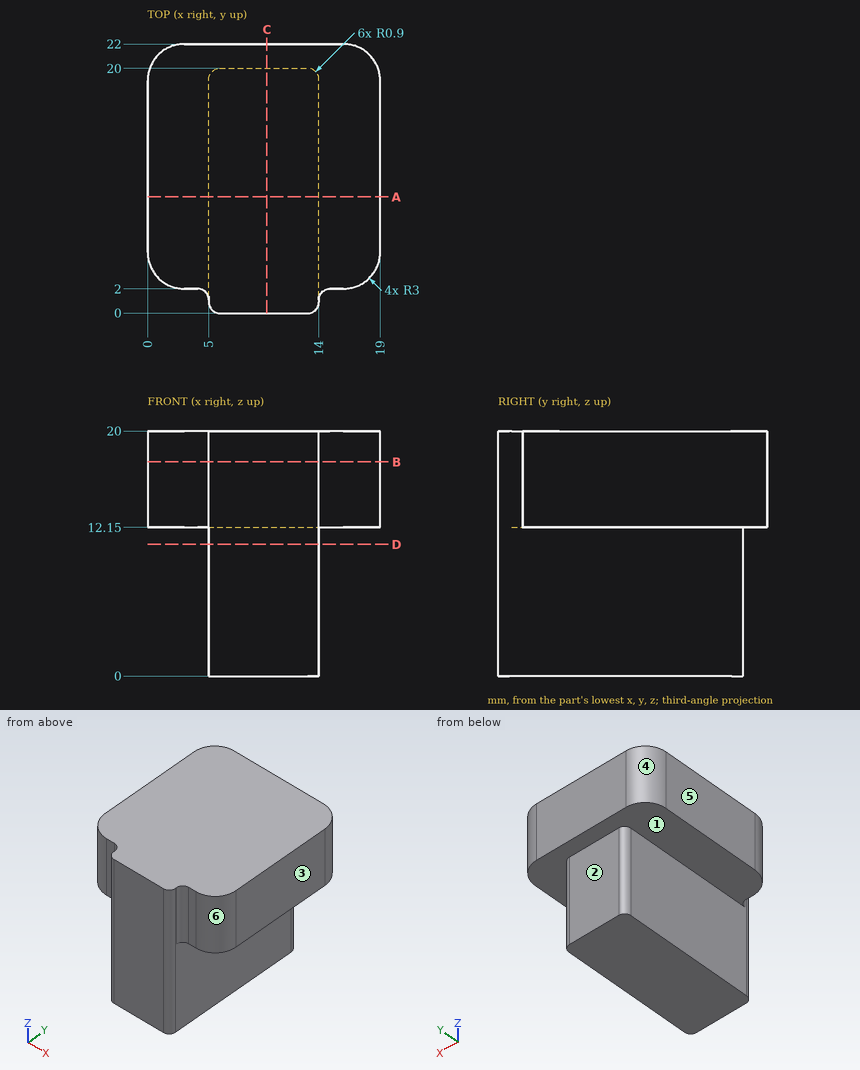
Part print with two shaded views. Sizes in mm from the minimum x, y, z corner. A direction names the side the tool comes from. Round coordinates to 2 decimals unless told otherwise and drop trailing zeros. Write each loop counter-clockwise with the first axis right and the second up, starting at its lowest first coordinate (ties: lowest second). Pieces come first, ordered by that corner, then holes. Notation, with made-up numbers: (79, -21.5) - (126, -21.5) arc R23 ccw to (126, -7.5) - close; hole circle Ø10 at (-1.75, 19). An arc over 180 degrees is marked (long way). Use CSV: the item, a comma, the result in double quotes.
Item 1: Tool access for the marked faces 1, 2 and 3: list every direction of +Z, -Z, +X, -X, +Y, -Y with a clear straight run to the whole face (end or side of a thin tool).
Results list:
face 1,"-Z, +Y"
face 2,"-Z, +X, -X, +Y"
face 3,"+Z, -Z, +X, +Y, -Y"
Item 2: Slice it at D-D, the plane z = 10.75. Write the cut outline in (x, y), then the cut area to 3 significant figures.
Results list:
outline,"(5, 0.9) arc R0.9 ccw to (5.9, 0) - (13.1, 0) arc R0.9 ccw to (14, 0.9) - (14, 19.1) arc R0.9 ccw to (13.1, 20) - (5.9, 20) arc R0.9 ccw to (5, 19.1) - close"
area,"179 mm²"
Item 3: Pull direction Y, two halves, no side cores. Call the marked faces 4, 5 and 6: pulls with the +Y half, pulls with the -Y half, needs draft (parallel to the pull), parting line crosses it, or undercut.
Results list:
face 4,"pulls with the +Y half"
face 5,"needs draft"
face 6,"pulls with the -Y half"
Item 4: Wall check: L1, parallel to X at y = 2.5, z = 6; L2, parallel to Y at x = 15, z = 15; L3, parallel to Z at x = 4.25, y = 18.25. Give the ranges that are in metal, low to high.
Results list:
L1,"x = 5 to 14"
L2,"y = 2 to 22"
L3,"z = 12.15 to 20"
Item 5: Slice it at A-A, the plane y = 9.5. Write the cut outline in (x, z).
Results list:
outline,"(0, 12.15) - (5, 12.15) - (5, 0) - (14, 0) - (14, 12.15) - (19, 12.15) - (19, 20) - (0, 20) - close"
Item 6: Slice it at C-C, the plane x = 9.75. Write the cut outline in (y, z).
Results list:
outline,"(0, 0) - (20, 0) - (20, 12.15) - (22, 12.15) - (22, 20) - (0, 20) - close"
Item 7: Slice it at B-B, the plane z = 17.5. Write the cut outline in (x, y), then the cut area to 3 significant figures.
Results list:
outline,"(0, 5) arc R3 ccw to (3, 2) - (4.1, 2) arc R0.9 cw to (5, 1.1) - (5, 0.9) arc R0.9 ccw to (5.9, 0) - (13.1, 0) arc R0.9 ccw to (14, 0.9) - (14, 1.1) arc R0.9 cw to (14.9, 2) - (16, 2) arc R3 ccw to (19, 5) - (19, 19) arc R3 ccw to (16, 22) - (3, 22) arc R3 ccw to (0, 19) - close"
area,"390 mm²"
Item 8: Flat gauge pins, fed straight in: P1, Ø3, axis at y = 10.5, z = 11, coming from the +X side; P2, Ø1.2, axis at x = 15.5, z = 16.5, coming from the -Y side; P3, Ø10, axis at y = 13, z = 6.5, coming from the +X side; P4, Ø4, axis at x = 4.5, z = 7, coming from the +Y side. Where does each tip first touch, or does it go through?
Results list:
P1,"stops at x = 19"
P2,"stops at y = 2"
P3,"stops at x = 14"
P4,"stops at y = 20"
